Geometry check sheet. Reference: the model listing, model coordinates, mm. A direction names the side the tool comes from. Coordinates: 2 decimals unless noted, no trailing zeros. Order: outer loops, then holes, each group sorted by start corner. A loop starts at its lowest first (then second) coordinate and runs counter-clockwise, first axis right, second up. Notation, with made-up numbers: M 62,55 L 100,55 A25 ccw 100,90 Z; hole C 66,1.5 d11. An arc over 180 degrees is marked long. One line per item, written item: value. Start each with the question number.
1) Draft check along Y on faces 1 (the cylindrical face through (4.388, 10.181, -13.812)), 2 (the flat face through (-1, 57, 0)), 3 (the flat face through (0, 53, 0)). Enter one of: pulls with the +Y half, pulls with the -Y half, needs draft (parallel to the pull), parting line crosses it, or undercut.
2) Sectioned sample at C-C, the plane y = 30. Enter the section's corners in (x, z).
3) Go/stop test with flat-tipped pins: P1, Ø7.5, axis at x = 0, y = 12, coming from the +Z side; P2, Ø8, axis at x = 10, y = 33, coming from the -Z side; P3, Ø1, axis at x = -0.5, z = -9.5, coming from the -Y side; P4, Ø10, axis at x = 7.5, y = 86, coming from the +Z side. Record where each tip stops, or that it passes through.
4) Access from +Z, -Z, +X, -X, +Y, -Y to the whole of each face (thin tool, end or side, straight path). Record for faces 4 (the cylindrical face through (-3.618, 78.801, -0.118)), 5 (the cylindrical face through (-4.788, 26.129, -11.547)), 6 (the flat face through (3, 100, 0)).
5) Sectioned sample at A-A, the plane y = 12. Enter the section's corners in (x, z), then the cut area to 3 significant figures.
6) Sectioned sample at B-B, the plane x = 0. State how many separate pieces and enclosed holes the cut face has, then the cut area to 3 significant figures.
7) Thickness scan on L1, parallel to X at y = 42, z = 0; L2, parallel to Z at x = -0.5, y = 49; L3, parallel to Y at x = 0, z = 13.25. Record the ranges inside material, lowest first. Write a range as from..to.
```python
from build123d import *

# Parameters (mm, degrees)
CUT_EXTRUDE1_DEPTH      = 103.528044944
CUT_EXTRUDE1_DEPTH_BACK = 103.528044944
SKETCH2_R               = 4.75
SKETCH3_R               = 12.5
CUT_EXTRUDE2_DEPTH      = 53
CUT_EXTRUDE3_DEPTH      = 43
FILLET1_R               = 5
FILLET2_R               = 3
FILLET3_R               = 3.5


with BuildPart() as part:
    # Sketch1 → Revolve1 (revolve)
    with BuildSketch(Plane(origin=(0, 0, 0), x_dir=(0, 0, -1), z_dir=(1, 0, 0)), mode=Mode.PRIVATE) as revolve1_sk:
        with BuildLine():
            Line((0, 0), (-16, 0))
            Line((-16, 0), (-16, 60))
            ThreePointArc((-16, 60), (-9.636038969, 62.636038969), (-7, 69))
            Line((-7, 69), (-7, 80))
            Line((-7, 80), (-7, 100))
            Line((-7, 100), (0, 100))
            Line((0, 100), (0, 0))
        make_face()
    revolve(revolve1_sk.sketch.rotate(Axis((0, 2.411465541, 0), (0, 1, 0)), 180), axis=Axis((0, 2.411465541, 0), (0, 1, 0)))

    # Sketch2 → Cut-Extrude1 (cut, two sides: drawn at the far end of the back side and taken through both)
    with BuildSketch(Plane.XY.offset(-CUT_EXTRUDE1_DEPTH_BACK)):
        with Locations((0, 12)):
            Circle(SKETCH2_R)
    extrude(amount=CUT_EXTRUDE1_DEPTH + CUT_EXTRUDE1_DEPTH_BACK, mode=Mode.SUBTRACT)

    # Sketch3 → Cut-Extrude2 (cut)
    with BuildSketch(Plane.XZ):
        with Locations(Location((0, 0, 0), (0, 0, 270))):
            Circle(SKETCH3_R)
    extrude(amount=-CUT_EXTRUDE2_DEPTH, mode=Mode.SUBTRACT)

    # Sketch4 → Cut-Extrude3 (cut)
    with BuildSketch(Plane(origin=(0, 100, 0), x_dir=(1, 0, 0), z_dir=(0, 1, 0))):
        with BuildLine():
            Line((2.4765, -2.639645431), (2.4765, 2.639645431))
            ThreePointArc((2.4765, 2.639645431), (-3.6195, 0), (2.4765, -2.639645431))
        make_face()
    extrude(amount=-CUT_EXTRUDE3_DEPTH, mode=Mode.SUBTRACT)

    # Fillet1
    fillet1_edges = [part.edges().sort_by_distance(p)[0] for p in [
        (0, 60, 16),
    ]]
    fillet(fillet1_edges, radius=FILLET1_R)

    # Fillet2
    fillet2_edges = [part.edges().sort_by_distance(p)[0] for p in [
        (0, 100, 7),
    ]]
    fillet(fillet2_edges, radius=FILLET2_R)

    # Fillet3
    fillet3_edges = [part.edges().sort_by_distance(p)[0] for p in [
        (0, 0, 16),
    ]]
    fillet(fillet3_edges, radius=FILLET3_R - 0.0001)  # a hair under: the kernel refuses the full size


solid = part.part
```
Final values:
1. face 1: undercut
1. face 2: pulls with the +Y half
1. face 3: pulls with the -Y half
2. outline: C 0,0 d32; hole C 0,0 d25
3. P1: passes through
3. P2: stops at z = -14.83
3. P3: stops at y = 53
3. P4: stops at z = 6.54
4. face 4: +Y
4. face 5: -Y
4. face 6: +Z, -Z, +X, -X, +Y
5. outline: M -4.75,-15.28 L -4.75,-11.56 A12.5 cw -4.75,11.56 L -4.75,15.28 A16 ccw Z; M 4.75,-15.28 A16 ccw 4.75,15.28 L 4.75,11.56 A12.5 cw 4.75,-11.56 Z
5. area: 246 mm^2
6. separate pieces: 3
6. enclosed holes: 0
6. area: 797 mm^2
7. L1: x = -16..-12.5, 12.5..16
7. L2: z = -15.99..-12.49, 12.49..15.99
7. L3: y = 0.08..7.25, 16.75..60.39
